The model under review builds one solid part; all positions refer to its coordinate system, in mm. Face numbers are marked on the shaded views. A direction names the side the tool comes from. Give positions to 0.01 mm unless a question says otherwise; leave off trailing zeros. Order: outer loops, then holes, each group sorted by start corner. A loop starts at its lowest first (then second) coordinate and runs counter-clockwise, first axis right, second up.
```python
from build123d import *

# Parameters (mm, degrees)
ESQUISSE1_R             = 12.5
ESQUISSE1_R_2           = 2
BOSS_EXTRU_1_DEPTH      = 16
ESQUISSE2_R             = 16.293222759
ESQUISSE2_R_2           = 2
BOSS_EXTRU_2_DEPTH      = 4
ESQUISSE3_R             = 3.5
ENL_V_MAT_EXTRU_1_DEPTH = 4
ESQUISSE4_W             = 7.413554481
ESQUISSE4_H             = 4
BOSS_EXTRU_3_DEPTH      = 4
CONG_1_R                = 2
CONG_2_R                = 0.4
ESQUISSE5_R             = 2.75
ENL_V_MAT_EXTRU_2_DEPTH = 5


with BuildPart() as part:
    # Esquisse1 → Boss.-Extru.1 (new body)
    with BuildSketch(Plane.XY):
        Circle(ESQUISSE1_R)
        Circle(ESQUISSE1_R_2, mode=Mode.SUBTRACT)
    extrude(amount=BOSS_EXTRU_1_DEPTH)

    # Esquisse2 → Boss.-Extru.2 (add)
    with BuildSketch(Plane.XY.offset(16)):
        Circle(ESQUISSE2_R)
        Circle(ESQUISSE2_R_2, mode=Mode.SUBTRACT)
    extrude(amount=BOSS_EXTRU_2_DEPTH)

    # Esquisse3 → Enlèv. mat.-Extru.1 (cut)
    with BuildSketch(Plane.XY.offset(20)):
        Circle(ESQUISSE3_R)
    extrude(amount=-ENL_V_MAT_EXTRU_1_DEPTH, mode=Mode.SUBTRACT)

    # Esquisse4 → Boss.-Extru.3 (add)
    with BuildSketch(Plane.XY.offset(20)):
        with Locations((16.29322276, 0)):
            Rectangle(ESQUISSE4_W, ESQUISSE4_H)
    extrude(amount=-BOSS_EXTRU_3_DEPTH)

    # Congé1
    cong_1_edges = [part.edges().sort_by_distance(p)[0] for p in [
        (16.170006428, -2, 18),
        (16.170006428, 2, 18),
    ]]
    fillet(cong_1_edges, radius=CONG_1_R)

    # Congé2
    cong_2_edges = [part.edges().sort_by_distance(p)[0] for p in [
        (20, -2, 18),
        (20, 2, 18),
    ]]
    fillet(cong_2_edges, radius=CONG_2_R)

    # Esquisse5 → Enlèv. mat.-Extru.2 (cut)
    with BuildSketch(Plane(origin=(0, 0, 0), x_dir=(-1, 0, 0), z_dir=(0, 0, -1))):
        with Locations((-6, 0)):
            Circle(ESQUISSE5_R)
        with Locations((3, 5.196152423)):
            Circle(ESQUISSE5_R)
        with Locations((3, -5.196152423)):
            Circle(ESQUISSE5_R)
    extrude(amount=-ENL_V_MAT_EXTRU_2_DEPTH, mode=Mode.SUBTRACT)


solid = part.part
```
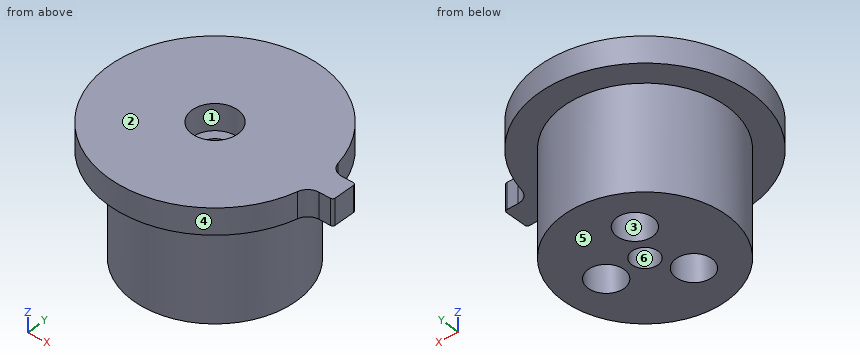
1. Take a section at B-B (x = 6). Write out the cut boundary in (y, z).
2. To check wall thickness, follow line 1 (Y direction, x = 0, z = 18.8); line 2 (X direction, y = 0.5, z = 3); line 3 (Z direction, x = -5.5, y = -6). State the ranges of each line that lie inside material, in increasing order.
3. Insertion check: pin 1 (2 mm diameter, centred on x = 7, y = -0.5, fed in from -Z); pin 2 (5.5 mm diameter, centred on x = 0, y = 0, fed in from +Z); pin 3 (6 mm diameter, centred on x = 7, z = 11, fed in from +Y). Each pin has a flat end and moves straight along its axis. Give the tip position at first contact, or say it passes through.
4. Take a section at D-D (z = 15.25). Write out the cut boundary in (x, y), and give its area (3 significant figures).
5. Take a section at A-A (y = 0). Write out the cut boundary in (x, z), and give its area (3 significant figures).
6. Draft analysis for pull direction Y (two halves, no side actions). For the marked faces 4, 5 and 6, state which applies: pulls with the +Y half, pulls with the -Y half, needs draft (parallel to the pull), parting line crosses it, or undercut.
7. For the marked faces 1, 2 and 3, list the 3-axis set-ups (+Z, -Z, +X, -X, +Y, -Y) from which the entire face can be reached by the end or side of a thin tool; tool diameter is ignored.
8. Take a section at C-C (y = -6). Write out the cut boundary in (x, z), and give its area (3 significant figures).
Answer:
1. outline: (-15.15, 16) - (-10.97, 16) - (-10.97, 0) - (-2.75, 0) - (-2.75, 5) - (2.75, 5) - (2.75, 0) - (10.97, 0) - (10.97, 16) - (15.15, 16) - (15.15, 20) - (-15.15, 20) - close
2. line 1: y = -16.29 to -3.5, 3.5 to 16.29
2. line 2: x = -12.49 to -1.94, 1.94 to 3.3, 8.7 to 12.49
2. line 3: z = 5 to 20
3. pin 1: stops at z = 5
3. pin 2: stops at z = 16
3. pin 3: stops at y = 11.84
4. outline: circle Ø25 at (0, 0); hole circle Ø4 at (0, 0)
4. area: 478 mm2
5. outline: (-16.29, 16) - (-12.5, 16) - (-12.5, 0) - (-2, 0) - (-2, 16) - (-3.5, 16) - (-3.5, 20) - (-16.29, 20) - close; (2, 0) - (3.25, 0) - (3.25, 5) - (8.75, 5) - (8.75, 0) - (12.5, 0) - (12.5, 16) - (20, 16) - (20, 20) - (3.5, 20) - (3.5, 16) - (2, 16) - close
5. area: 426 mm2
6. face 4: parting line crosses it
6. face 5: needs draft
6. face 6: undercut
7. face 1: +Z
7. face 2: +Z, +X, -X, +Y, -Y
7. face 3: -Z
8. outline: (-15.15, 16) - (-10.97, 16) - (-10.97, 0) - (-5.63, 0) - (-5.63, 5) - (-0.37, 5) - (-0.37, 0) - (10.97, 0) - (10.97, 16) - (15.15, 16) - (15.15, 20) - (-15.15, 20) - close
8. area: 446 mm2
